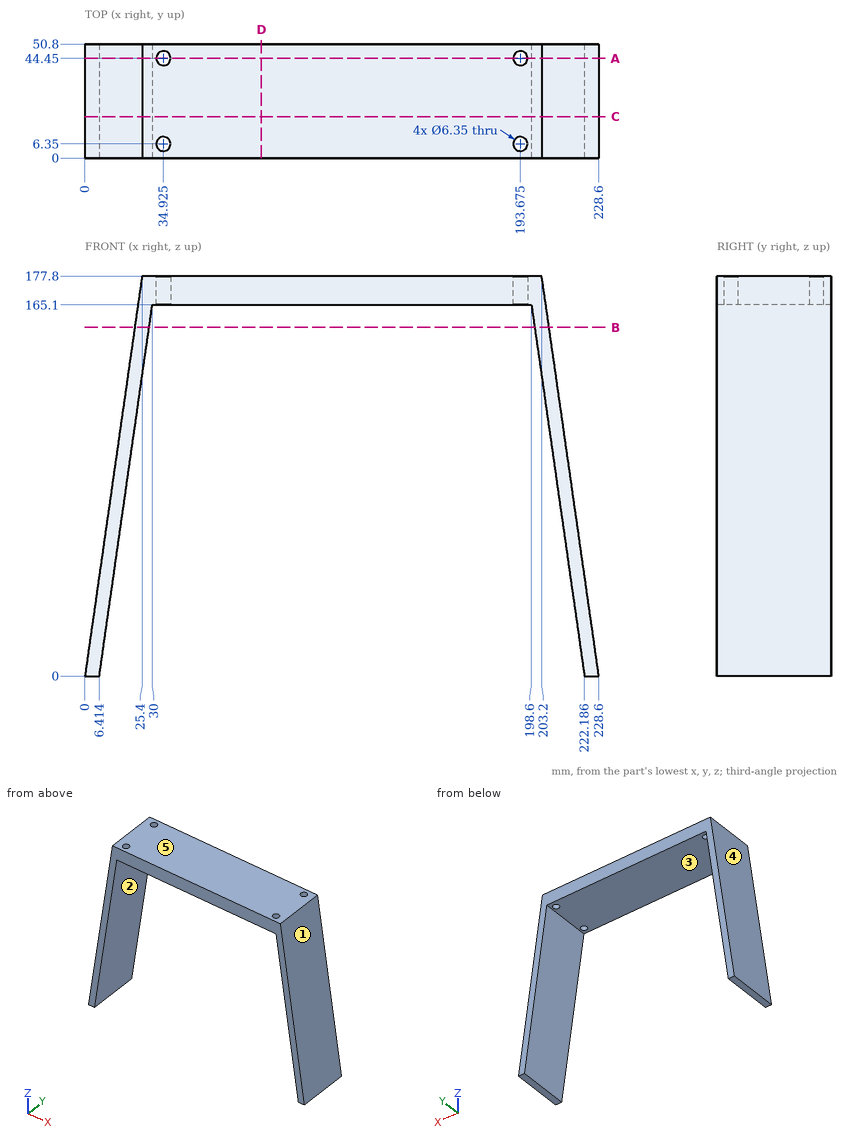
Can you work these out from the drawing? Everything is in mm from the part's minimum corner. A direction names the side the tool comes from. Give positions to 0.01 mm unless a question says otherwise; leave off trailing zeros. Loops run counter-clockwise (first coordinate to the right, second up) from the corner with the lowest first, then second, coordinate; pieces in that order, holes last. Notation, with made-up numbers: (19.5, -32) -> (35.5, -32) arc R6 ccw to (35.5, -26) -> close; hole circle Ø1 at (-25, 86.25). An arc over 180 degrees is marked (long way). Return JSON: item names as keys, results as strings.
Q1. I want a section at C-C, the plane y = 18.5. List the corners of the cut face in (x, z) for me (1 decimal), then the cut area to 3 significant figures.
Checks:
{"outline": "(0, 0) -> (6.4, 0) -> (30, 165.1) -> (198.6, 165.1) -> (222.2, 0) -> (228.6, 0) -> (203.2, 177.8) -> (25.4, 177.8) -> close", "area": "4,400 mm2"}
Q2. I want a section at D-D, the plane x = 78.5. List the corners of the cut face in (y, z) for me, then the cut area to 3 significant figures.
Checks:
{"outline": "(0, 165.1) -> (50.8, 165.1) -> (50.8, 177.8) -> (0, 177.8) -> close", "area": "645 mm2"}
Q3. I want a section at B-B, the plane z = 155. List the corners of the cut face in (x, y) for me.
Checks:
{"outline": "(22.14, 0) -> (28.56, 0) -> (28.56, 50.8) -> (22.14, 50.8) -> close; (200.04, 0) -> (206.46, 0) -> (206.46, 50.8) -> (200.04, 50.8) -> close"}
Q4. For pin 1 Ø2 at (y, z) = (13.5, 107.5) entering from -X; pin 2 Ø4 at (x, y) = (193.675, 6.35) entering from -Z; pin 3 Ø4 at (y, z) = (20, 46) entering from +X; pin 4 Ø1.5 at (x, y) = (118.5, 23.5) entering from -Z, each with a flat end and sliding along its axis, tell me the tip position at first contact or that it passes through.
Checks:
{"pin 1": "stops at x = 15.21", "pin 2": "passes through", "pin 3": "stops at x = 222.31", "pin 4": "stops at z = 165.1"}
Q5. I need wall thicknesses on probe 1 along Y at (x, z) = (33, 170) (1 decimal); probe 2 along X at (y, z) = (6, 173) (1 decimal); probe 3 along X at (y, z) = (6, 169). Which ranges of each line are inside material? Lowest first, please.
Checks:
{"probe 1": "y = 0 to 3.8, 8.9 to 41.9, 47 to 50.8", "probe 2": "x = 24.7 to 31.8, 38.1 to 190.5, 196.8 to 203.9", "probe 3": "x = 24.14 to 31.77, 38.08 to 190.52, 196.83 to 204.46"}
Q6. I want a section at A-A, the plane y = 44.45. Count the separate pieces of the cut face and the enclosed holes in it, then the cut area to 3 significant figures.
Checks:
{"separate pieces": "3", "enclosed holes": "0", "area": "4,240 mm2"}
Q7. We'd pull the mould along X, two halves only. Please class the marked faces 3, 4 and 5: released by +X, released by -X, zero draft, split by the parting line, or undercut.
Checks:
{"face 3": "undercut", "face 4": "released by -X", "face 5": "zero draft"}
Q8. On a 3-axis mill with a long thin cutter (end or side, diameter ignored), from which of +Z, -Z, +X, -X, +Y, -Y can I reach the whole of each face in a straight line? I mean the marked faces 1 and 2. Say none if no direction works.
Checks:
{"face 1": "+Z, +X, +Y, -Y", "face 2": "-Z, +Y, -Y"}
